Can you work these out from the model? Positions are in its coordinate system, mm. A direction names the side the tool comes from. Coordinates: 2 decimals unless noted, no trailing zeros. Loops run counter-clockwise (first coordinate to the right, second up) from the corner with the lowest first, then second, coordinate; pieces in that order, holes last.
```python
from build123d import *

# Parameters (mm, degrees)
SKETCH_1_W          = 38.5
SKETCH_1_H          = 102.6
EXTRUDE_1_DEPTH     = 2
SKETCH_2_R          = 1.6
CUT_EXTRUDE_1_DEPTH = 2
SKETCH_3_W          = 80
SKETCH_3_H          = 36
EXTRUDE_2_DEPTH     = 2
SKETCH_4_R          = 1.6
SKETCH_4_W          = 28.5
SKETCH_4_H          = 55.6
SKETCH_4_W_2        = 102.60113133
SKETCH_4_H_2        = 28
CUT_EXTRUDE_2_DEPTH = 10
EXTRUDE_START       = -2
EXTRUDE_2_2_DEPTH   = 2
FILLET_1_R          = 2
FILLET_2_R          = 2


# Read off the part's stored shape, not the designer's step: 拉伸-薄壁2
with BuildPart() as part:
    # 草图1 → 凸台-拉伸1 (new body)
    with BuildSketch(Plane(origin=(0, 0, 0), x_dir=(1, 0, 0), z_dir=(0, 1, 0))):
        Rectangle(SKETCH_1_W, SKETCH_1_H)
    extrude(amount=EXTRUDE_1_DEPTH)

    # 草图2 → 切除-拉伸1 (cut)
    with BuildSketch(Plane(origin=(0, 2, 0), x_dir=(1, 0, 0), z_dir=(0, 1, 0))):
        with Locations(Location((-16.25, -46.3, 0), (0, 0, 270))):
            Circle(SKETCH_2_R)
        with Locations(Location((16.25, -46.3, 0), (0, 0, 270))):
            Circle(SKETCH_2_R)
        with Locations(Location((-16.25, 22.3, 0), (0, 0, 270))):
            Circle(SKETCH_2_R)
        with Locations(Location((-16.25, 46.3, 0), (0, 0, 270))):
            Circle(SKETCH_2_R)
    extrude(amount=-CUT_EXTRUDE_1_DEPTH, mode=Mode.SUBTRACT)

    # 草图3 → Extrude 2 (add)
    with BuildSketch(Plane(origin=(0, 2, 0), x_dir=(1, 0, 0), z_dir=(0, 1, 0))):
        with Locations((59.25, 33.3)):
            Rectangle(SKETCH_3_W, SKETCH_3_H)
    extrude(amount=-EXTRUDE_2_DEPTH)

    # 草图4 → 切除-拉伸2 (cut)
    with BuildSketch(Plane(origin=(0, 2, 0), x_dir=(1, 0, 0), z_dir=(0, 1, 0))):
        with Locations(Location((94.75, 46.3, 0), (0, 0, 270))):
            Circle(SKETCH_4_R)
        with Locations(Location((94.75, 22.3, 0), (0, 0, 270))):
            Circle(SKETCH_4_R)
        with Locations(Location((-16.25, 22.3, 0), (0, 0, 270))):
            Circle(SKETCH_4_R)
        with Locations(Location((-16.25, 46.3, 0), (0, 0, 270))):
            Circle(SKETCH_4_R)
        with Locations((0, -14.5)):
            Rectangle(SKETCH_4_W, SKETCH_4_H)
        with Locations((39.050565665, 33.3)):
            Rectangle(SKETCH_4_W_2, SKETCH_4_H_2)
    extrude(amount=-CUT_EXTRUDE_2_DEPTH, mode=Mode.SUBTRACT)

    # Extrude 2 2 outline → Extrude 2 2 (add)
    # profile 1 of 6: a face of its own
    with BuildSketch(Plane(origin=(0, 2, 0), x_dir=(1, 0, 0), z_dir=(0, 1, 0)).offset(EXTRUDE_START)):
        Polygon((21.873623978, 35.651249756), (10.224873734, 47.3), (5.275126266, 47.3), (33.275126266, 19.3), (44.826005064, 19.3), (72.826005064, 47.3), (67.876257596, 47.3), (56.227507352, 35.651249756), (41.832509602, 47.3), (36.268621728, 47.3), align=None)
        Polygon((37.300565665, 20.224308069), (24.362218946, 33.162654788), (37.300565665, 43.632650831), align=None, mode=Mode.SUBTRACT)
        Polygon((40.800565665, 43.632650831), (53.738912383, 33.162654788), (40.800565665, 20.224308069), align=None, mode=Mode.SUBTRACT)
    # profile 2 of 6: a face of its own
    with BuildSketch(Plane(origin=(0, 2, 0), x_dir=(1, 0, 0), z_dir=(0, 1, 0)).offset(EXTRUDE_START)):
        Polygon((18.224873734, 19.3), (-9.775126266, 47.3), (-12.25, 47.3), (-12.25, 44.825126266), (13.275126266, 19.3), align=None)
    # profile 3 of 6: a face of its own
    with BuildSketch(Plane(origin=(0, 2, 0), x_dir=(1, 0, 0), z_dir=(0, 1, 0)).offset(EXTRUDE_START)):
        Polygon((87.876257596, 47.3), (59.876257596, 19.3), (64.826005064, 19.3), (90.35113133, 44.825126266), (90.35113133, 47.3), align=None)
    # profile 4 of 6: a face of its own
    with BuildSketch(Plane(origin=(0, 2, 0), x_dir=(1, 0, 0), z_dir=(0, 1, 0)).offset(EXTRUDE_START)):
        Polygon((-0.724873734, 19.3), (4.224873734, 19.3), (-12.25, 35.774873734), (-12.25, 30.825126266), align=None)
    # profile 5 of 6: a face of its own
    with BuildSketch(Plane(origin=(0, 2, 0), x_dir=(1, 0, 0), z_dir=(0, 1, 0)).offset(EXTRUDE_START)):
        Polygon((90.35113133, 35.774873734), (73.876257596, 19.3), (78.826005064, 19.3), (90.35113133, 30.825126266), align=None)
    # profile 6 of 6: a face of its own
    with BuildSketch(Plane(origin=(0, 2, 0), x_dir=(1, 0, 0), z_dir=(0, 1, 0)).offset(EXTRUDE_START)):
        Polygon((-14.25, 13.3), (-14.25, 9.463577763), (-1.966511398, -14.5), (-14.25, -38.463577763), (-14.25, -42.3), (-12.283488602, -42.3), (0, -18.336422237), (12.283488602, -42.3), (14.25, -42.3), (14.25, -38.463577763), (1.966511398, -14.5), (14.25, 9.463577763), (14.25, 13.3), (12.283488602, 13.3), (0, -10.663577763), (-12.283488602, 13.3), align=None)
    extrude(amount=EXTRUDE_2_2_DEPTH)

    # 圆角1
    fillet_1_edges = [part.edges().sort_by_distance(p)[0] for p in [
        (44.826005064, 1, -19.3),
        (33.275126266, 1, -19.3),
        (36.268621728, 1, -47.3),
        (67.876257596, 1, -47.3),
        (41.832509602, 1, -47.3),
        (10.224873734, 1, -47.3),
        (21.873623978, 1, -35.651249756),
        (56.227507352, 1, -35.651249756),
        (5.275126266, 1, -47.3),
        (72.826005064, 1, -47.3),
        (37.300565665, 1, -20.224308069),
        (40.800565665, 1, -43.632650831),
        (40.800565665, 1, -20.224308069),
        (53.738912383, 1, -33.162654788),
        (24.362218946, 1, -33.162654788),
        (37.300565665, 1, -43.632650831),
        (90.35113133, 1, -30.825126266),
        (90.35113133, 1, -35.774873734),
        (73.876257596, 1, -19.3),
        (78.826005064, 1, -19.3),
        (90.35113133, 1, -44.825126266),
        (87.876257596, 1, -47.3),
        (64.826005064, 1, -19.3),
        (59.876257596, 1, -19.3),
        (18.224873734, 1, -19.3),
        (13.275126266, 1, -19.3),
        (-12.25, 1, -44.825126266),
        (-9.775126266, 1, -47.3),
        (4.224873734, 1, -19.3),
        (-0.724873734, 1, -19.3),
        (-12.25, 1, -30.825126266),
        (-12.25, 1, -35.774873734),
        (-12.283488602, 1, 42.3),
        (12.283488602, 1, 42.3),
        (14.25, 1, -9.463577763),
        (14.25, 1, 38.463577763),
        (12.283488602, 1, -13.3),
        (-12.283488602, 1, -13.3),
        (-14.25, 1, 38.463577763),
        (-14.25, 1, -9.463577763),
        (-1.966511398, 1, 14.5),
        (0, 1, 10.663577763),
        (1.966511398, 1, 14.5),
        (0, 1, 18.336422237),
        (-12.25, 1, -19.3),
        (90.35113133, 1, -19.3),
    ]]
    fillet(fillet_1_edges, radius=FILLET_1_R)

    # 圆角2
    fillet_2_edges = [part.edges().sort_by_distance(p)[0] for p in [
        (19.25, 1, -15.3),
        (99.25, 1, -51.3),
        (99.25, 1, -15.3),
        (19.25, 1, 51.3),
        (-19.25, 1, 51.3),
        (-19.25, 1, -51.3),
    ]]
    fillet(fillet_2_edges, radius=FILLET_2_R)


solid = part.part
```
(1) I'm going to push a flat-ended pin straight in: pin 1 (1 mm diameter, centred on y = 1.5, z = 21.5, fed in from +X). Where does the tip first touch, or does it pass through?
Check values:
pin 1: stops at x = 19.25
(2) I want a section at D-D on y = 0.95. State how many separate pieces and enclosed holes the cut face has, then the cut area to 3 significant figures.
Check values:
separate pieces: 1
enclosed holes: 20
area: 3,810 mm2
(3) Which directions (+Z, -Z, +X, -X, +Y, -Y) give clear straight access to the entire face, cutting with the end or side of a thin tool? Please do faces 3 (the flat face through (6.348, 0.986, -1.721)), 4 (the flat face through (31, 2, -19)).
Check values:
face 3: +Y, -Y
face 4: +Z, -Z, +X, -X, +Y
(4) I want a section at B-B on x = 94.75. Write out the boundary of the cut face in (y, z), then the cut area to 3 significant figures.
Check values:
outline: (0, -51.3) - (2, -51.3) - (2, -47.9) - (0, -47.9) - close; (0, -44.7) - (2, -44.7) - (2, -23.9) - (0, -23.9) - close; (0, -20.7) - (2, -20.7) - (2, -15.3) - (0, -15.3) - close
area: 59.2 mm2
(5) If we mould it in two halves opening along X, with no side actions, what happens to faces 1 (the flat face through (31, 0, -19)), 2 (the flat face through (60.072, 0.986, -34.546))? For each: released by +X, released by -X, zero draft, split by the parting line, or undercut.
Check values:
face 1: zero draft
face 2: undercut
(6) If I drill on probe 1 along X at (y, z) = (0.55, 46.3); probe 2 along Z at (x, y) = (94.75, 1.2); probe 3 along Z at (x, y) = (77, 1.5), over which ranges is the centre line in solid material (lowest first)?
Check values:
probe 1: x = -19.25 to -17.85, -14.65 to 14.65, 17.85 to 19.25
probe 2: z = -51.3 to -47.9, -44.7 to -23.9, -20.7 to -15.3
probe 3: z = -51.3 to -47.3, -36.42 to -31.47, -22.42 to -15.3
(7) I want a section at C-C on z = -30. Write out the boundary of the cut face in (x, y), then the cut area to 3 significant figures.
Check values:
outline: (-19.25, 0) - (-6.48, 0) - (-6.48, 2) - (-19.25, 2) - close; (2.58, 0) - (7.52, 0) - (7.52, 2) - (2.58, 2) - close; (22.58, 0) - (27.52, 0) - (27.52, 2) - (22.58, 2) - close; (37.3, 0) - (40.8, 0) - (40.8, 2) - (37.3, 2) - close; (50.58, 0) - (55.53, 0) - (55.53, 2) - (50.58, 2) - close; (70.58, 0) - (75.53, 0) - (75.53, 2) - (70.58, 2) - close; (84.58, 0) - (99.25, 0) - (99.25, 2) - (84.58, 2) - close
area: 101 mm2
(8) I want a section at A-A on z = 46.3. Write out the boundary of the cut face in (x, y).
Check values:
outline: (-19.25, 0) - (-17.85, 0) - (-17.85, 2) - (-19.25, 2) - close; (-14.65, 0) - (14.65, 0) - (14.65, 2) - (-14.65, 2) - close; (17.85, 0) - (19.25, 0) - (19.25, 2) - (17.85, 2) - close
